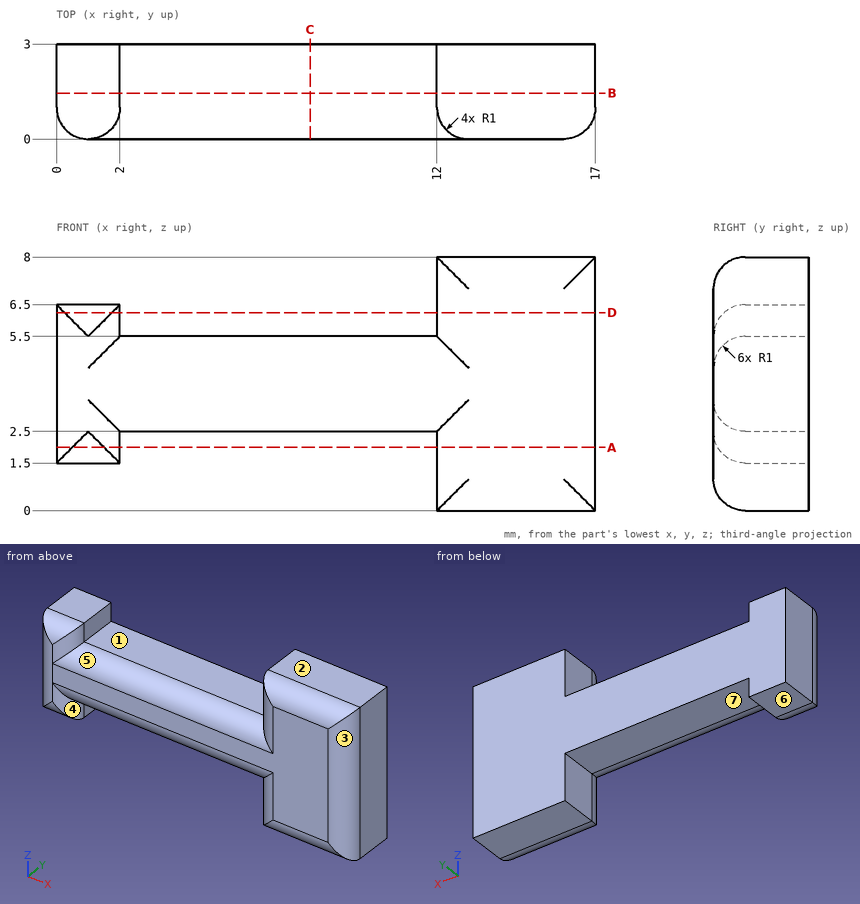
Answer from the drawing. Dimensions are ordinates in mm from the lowest x, y and z of the part. A direction names the side the tool comes from. Give positions to 0.01 mm unless a question says otherwise; leave off trailing zeros. Loops run counter-clockwise (first coordinate to the right, second up) from the corner with the lowest first, then second, coordinate; pieces in that order, holes last. Notation, with made-up numbers: (-14.75, 29.25) - (20.25, 29.25) arc R15 cw to (20.25, 45.25) - close; hole circle Ø3 at (-6.75, 63.5). An arc over 180 degrees is marked (long way). Write each question's results on one line, items separated by ' | '.
1. Find section C-C, the plane x = 8. Write down the section's boundary in (y, z).
Resolved:
outline: (0, 3.5) arc R1 ccw to (1, 2.5) - (3, 2.5) - (3, 5.5) - (1, 5.5) arc R1 ccw to (0, 4.5) - close
2. Find section A-A, the plane z = 2. Write down the section's boundary in (x, y).
Resolved:
outline: (0, 1) arc R1 ccw to (0.5, 0.13) - (1.5, 0.13) arc R1 ccw to (2, 1) - (2, 3) - (0, 3) - close; (12, 1) arc R1 ccw to (13, 0) - (16, 0) arc R1 ccw to (17, 1) - (17, 3) - (12, 3) - close
3. Find section D-D, the plane z = 6.25. Write down the section's boundary in (x, y), then the cut area to 3 significant figures.
Resolved:
outline: (0, 1) arc R1 ccw to (0.25, 0.34) - (1.75, 0.34) arc R1 ccw to (2, 1) - (2, 3) - (0, 3) - close; (12, 1) arc R1 ccw to (13, 0) - (16, 0) arc R1 ccw to (17, 1) - (17, 3) - (12, 3) - close | area: 19.8 mm^2
4. For a pull along X with two mould halves and no side action, classify the marked faces 1, 2 and 3 as +X half, -X half, draft (parallel to the pull), parting line (faces both ways), or undercut.
Resolved:
face 1: undercut | face 2: draft | face 3: +X half
5. Which of the six approach directions +Z, -Z, +X, -X, +Y, -Y give full straight-line access (tool end or side, diameter ignored) to the marked faces 4, 5, 6 and 7?
Resolved:
face 4: -Z, -Y | face 5: +Z, -Y | face 6: -Z, -X, +Y, -Y | face 7: -Z, +Y, -Y
6. Find section B-B, the plane y = 1.45. Write down the section's boundary in (x, z), then the cut area to 3 significant figures.
Resolved:
outline: (0, 1.5) - (2, 1.5) - (2, 2.5) - (12, 2.5) - (12, 0) - (17, 0) - (17, 8) - (12, 8) - (12, 5.5) - (2, 5.5) - (2, 6.5) - (0, 6.5) - close | area: 80.0 mm^2
7. Flat-ended cylindrical pins translate along their axes: P1, Ø0.6, axis at x = 1.5, y = 1.5, coming from the +Z side; P2, Ø1, axis at x = 8.5, y = 1, coming from the -Z side; P3, Ø0.6, axis at x = 1, y = 2, coming from the -Z side. Find the tip coordinate at first contact, or state that the pin passes through.
Resolved:
P1: stops at z = 6.5 | P2: stops at z = 2.5 | P3: stops at z = 1.5
8. Consider probe 1 along X at (y, z) = (1.95, 1.75); probe 2 along X at (y, z) = (1.7, 7); probe 3 along Z at (x, y) = (9.5, 2.8). Determine where each line is inside the solid, lowest interval first. Write a range as from..to.
Resolved:
probe 1: x = 0..2, 12..17 | probe 2: x = 12..17 | probe 3: z = 2.5..5.5
